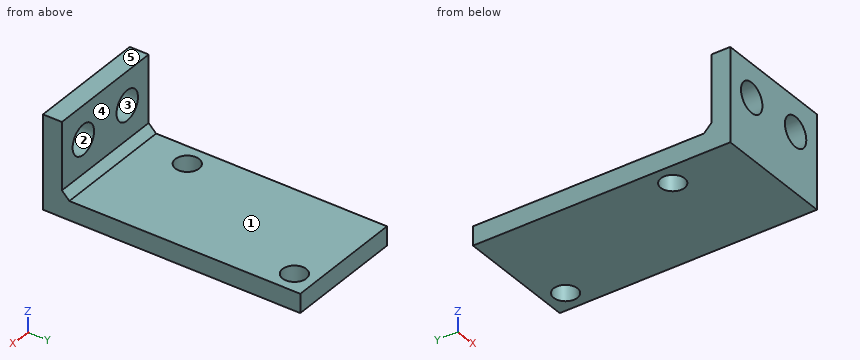
from build123d import *

# Parameters (mm, degrees)
SKETCH1_W           = 16.2
SKETCH1_H           = 34.54
BOSS_EXTRUDE1_DEPTH = 2.54
SKETCH2_W           = 16.2
SKETCH2_H           = 2.54
BOSS_EXTRUDE2_DEPTH = 10
CHAMFER1_SIZE       = 1
SKETCH4_R           = 1.6
CUT_EXTRUDE1_DEPTH  = 2.54
SKETCH5_R           = 2
CUT_EXTRUDE2_DEPTH  = 3.54


with BuildPart() as part:
    # Sketch1 → Boss-Extrude1 (new body)
    with BuildSketch(Plane.XY):
        with Locations((8.1, 17.27)):
            Rectangle(SKETCH1_W, SKETCH1_H)
    extrude(amount=BOSS_EXTRUDE1_DEPTH)

    # Sketch2 → Boss-Extrude2 (add)
    with BuildSketch(Plane.XY.offset(2.54)):
        with Locations((8.1, 1.27)):
            Rectangle(SKETCH2_W, SKETCH2_H)
    extrude(amount=BOSS_EXTRUDE2_DEPTH)

    # Chamfer1
    chamfer1_edges = [part.edges().sort_by_distance(p)[0] for p in [
        (8.1, 2.54, 2.54),
    ]]
    chamfer(chamfer1_edges, length=CHAMFER1_SIZE)

    # Sketch4 → Cut-Extrude1 (cut)
    with BuildSketch(Plane(origin=(0, 0, 0), x_dir=(-1, 0, 0), z_dir=(0, 0, -1))):
        with Locations((-13.4, 31.74)):
            Circle(SKETCH4_R)
        with Locations((-2.8, 9.74)):
            Circle(SKETCH4_R)
    extrude(amount=-CUT_EXTRUDE1_DEPTH, mode=Mode.SUBTRACT)

    # Sketch5 → Cut-Extrude2 (cut, through all)
    with BuildSketch(Plane(origin=(0, 2.54, 0), x_dir=(1, 0, 0), z_dir=(0, 1, 0))):
        with Locations((12.2, -8.04)):
            Circle(SKETCH5_R)
        with Locations((4, -8.04)):
            Circle(SKETCH5_R)
    extrude(amount=-CUT_EXTRUDE2_DEPTH, mode=Mode.SUBTRACT)


solid = part.part
Geometry check sheet. Reference: the model listing, model coordinates, mm. Face numbers are marked on the shaded views. A direction names the side the tool comes from. Round coordinates to 2 decimals unless told otherwise and drop trailing zeros. Order: outer loops, then holes, each group sorted by start corner. A loop starts at its lowest first (then second) coordinate and runs counter-clockwise, first axis right, second up. Notation, with made-up numbers: M 49,29.25 L 58,29.25 A6 cw 58,33.25 Z; hole C -15.5,77 d7. An arc over 180 degrees is marked long. Answer in a Markdown table with one row per item. Add a question column.
Item 1: Depth check by flat-ended pin: pin 1 Ø5 at (x, y) = (4, 25) entering from +Z; pin 2 Ø3.5 at (x, y) = (13.4, 31.74) entering from -Z; pin 3 Ø3.5 at (x, z) = (12.2, 8.04) entering from -Y; pin 4 Ø5 at (x, z) = (14, 8) entering from +Y. Enter the tip coordinate at first touch or a pass-through.
Item 2: Material ranges on L1, parallel to X at y = 1.95, z = 8.04; L2, parallel to Y at x = 2.8, z = 1.25; L3, parallel to Z at x = 6.5, y = 28.5, recorded low to high. Write a range as [from, to].
Item 3: Sectioned sample at D-D, the plane x = 4.75. Enter the section's corners in (y, z).
Item 4: Draft check along Z on the marked faces 3, 4 and 5. Enter one of: released by +Z, released by -Z, zero draft, split by the parting line, or undercut.
Item 5: Sectioned sample at C-C, the plane z = 8.04. Enter the section's corners in (x, y).
Item 6: Sectioned sample at B-B, the plane y = 9.74. Enter the section's corners in (x, z), plus the area to 3 significant figures.
Item 7: Sectioned sample at A-A, the plane x = 13.4. Enter the section's corners in (y, z).
Item 8: Set-up check for the marked faces 1 and 2: record each of +Z, -Z, +X, -X, +Y, -Y from which the full face is reachable in a straight line by a thin tool's end or side.
Filled in:
| question | item | result |
|---|---|---|
| 1 | pin 1 | stops at z = 2.54 |
| 1 | pin 2 | stops at z = 0 |
| 1 | pin 3 | passes through |
| 1 | pin 4 | stops at y = 2.54 |
| 2 | L1 | x = [0, 2], [6, 10.2], [14.2, 16.2] |
| 2 | L2 | y = [0, 8.14], [11.34, 34.54] |
| 2 | L3 | z = [0, 2.54] |
| 3 | outline | M 0,0 L 34.54,0 L 34.54,2.54 L 3.54,2.54 L 2.54,3.54 L 2.54,6.19 L 0,6.19 Z; M 0,9.89 L 2.54,9.89 L 2.54,12.54 L 0,12.54 Z |
| 4 | face 3 | undercut |
| 4 | face 4 | zero draft |
| 4 | face 5 | released by +Z |
| 5 | outline | M 0,0 L 2,0 L 2,2.54 L 0,2.54 Z; M 6,0 L 10.2,0 L 10.2,2.54 L 6,2.54 Z; M 14.2,0 L 16.2,0 L 16.2,2.54 L 14.2,2.54 Z |
| 6 | outline | M 0,0 L 1.2,0 L 1.2,2.54 L 0,2.54 Z; M 4.4,0 L 16.2,0 L 16.2,2.54 L 4.4,2.54 Z |
| 6 | area | 33.0 mm² |
| 7 | outline | M 0,0 L 30.14,0 L 30.14,2.54 L 3.54,2.54 L 2.54,3.54 L 2.54,6.44 L 0,6.44 Z; M 0,9.64 L 2.54,9.64 L 2.54,12.54 L 0,12.54 Z; M 33.34,0 L 34.54,0 L 34.54,2.54 L 33.34,2.54 Z |
| 8 | face 1 | +Z, +X, -X, +Y |
| 8 | face 2 | +Y, -Y |
